Part model, mm, in its own coordinate system. A direction names the side the tool comes from. Give positions to 0.01 mm unless a question says otherwise; leave off trailing zeros. Write each loop counter-clockwise with the first axis right and the second up, starting at its lowest first coordinate (ties: lowest second). Pieces come first, ordered by that corner, then holes. Notation, with made-up numbers: M 20.5,33 L 69.5,33 A20 cw 69.5,61 Z; hole C -29,-19 d1. An arc over 180 degrees is marked long. Use CSV: the item, a comma, the result in double quotes. Start each with the question number.
Item 1: Pin check, flat tips, straight feed: pin 1 (18 mm diameter, centred on x = 20.5, z = -3.5, fed in from +Y); pin 2 (4 mm diameter, centred on x = -7, z = -0.5, fed in from +Y); pin 3 (1.7 mm diameter, centred on x = -14.1, z = -4.95, fed in from +Y); pin 4 (10 mm diameter, centred on y = 17.5, z = -0.5, fed in from -X). Stop position of each tip, or through.
Item 2: Mould opens along Z. For faces 1 (the flat face through (39, 11, 23.5)), 2 (the flat face through (16, 11, -11.25)), 3 (the cylindrical face through (-23.494, 3.36, -0.517)) say: released by +Z, released by -Z, zero draft, split by the parting line, or undercut.
Item 3: Cut at B-B (y = 14.25). List the corners of the cut face in (x, z), then the cut area to 3 significant figures.
Item 4: Which spindle directions (+Z, -Z, +X, -X, +Y, -Y) get a long thin tool onto all of the face, cutting with end or side? Do faces 4 (the flat face through (16, 11, 11.25)), 5 (the cylindrical face through (35.57, 1.48, 3.97)). Say none if no direction does.
Item 5: Cut at C-C (z = -2.5). List the corners of the cut face in (x, y), then the cut area to 3 significant figures.
Item 6: Cut at A-A (x = 34.5). List the corners of the cut face in (y, z), then the cut area to 3 significant figures.
Item 7: Cut at D-D (y = 8.75). List the corners of the cut face in (x, z).
Item 8: Drill centre lines: line 1 (Z direction, x = 34.5, y = 1.25); line 2 (Z direction, x = 30, y = 15.25); line 3 (Y direction, x = 3.5, z = 7). Where is each one in solid material? Low to high. Write a range as [from, to].
from build123d import *

# Parameters (mm, degrees)
SKETCH1_R               = 23.5
SKETCH1_W               = 80
SKETCH1_H               = 47
BOSS_EXTRUDE1_DEPTH     = 23
SKETCH3_W               = 56
SKETCH3_H               = 22.5
CUT_EXTRUDE1_DEPTH      = 20
CUT_EXTRUDE2_DEPTH      = 48
M3_5X0_6_TAPPED_HOLE1_D = 2.9


with BuildPart() as part:
    # Sketch1 → Boss-Extrude1 (new body)
    with BuildSketch(Plane(origin=(0, 0, 0), x_dir=(1, 0, 0), z_dir=(0, 1, 0))):
        Circle(SKETCH1_R)
        with Locations((40, 0)):
            Rectangle(SKETCH1_W, SKETCH1_H)
    extrude(amount=BOSS_EXTRUDE1_DEPTH)

    # Sketch3 → Cut-Extrude1 (cut)
    with BuildSketch(Plane(origin=(0, 23, 0), x_dir=(1, 0, 0), z_dir=(0, 1, 0))):
        with Locations((10.2, 0)):
            Rectangle(SKETCH3_W, SKETCH3_H)
    extrude(amount=-CUT_EXTRUDE1_DEPTH, mode=Mode.SUBTRACT)

    # Sketch4 → Cut-Extrude2 (cut, through all)
    with BuildSketch(Plane.XY.offset(23.5)):
        with BuildLine():
            Line((0, 23), (29.574214856, 23))
            ThreePointArc((29.574214856, 23), (13.980947767, 19.955758133), (0, 12.409203517))
            ThreePointArc((0, 12.409203517), (-11.118700592, 6.831963759), (-23.5, 5.634244617))
            Line((-23.5, 5.634244617), (-23.5, 23))
            Line((-23.5, 23), (0, 23))
        make_face()
    extrude(amount=-CUT_EXTRUDE2_DEPTH, mode=Mode.SUBTRACT)

    # M3.5x0.6 Tapped Hole1 (through all)
    with Locations(Plane(origin=(0, 3, 0), x_dir=(1, 0, 0), z_dir=(0, 1, 0))):
        with Locations((-14.100375238, 4.953237367), (-14.100375238, -4.956255047), (34.5, -4.95), (34.5, 4.953237367)):
            Hole(M3_5X0_6_TAPPED_HOLE1_D / 2)


solid = part.part
Worked answers:
1,pin 1,"stops at y = 22.62"
1,pin 2,"stops at y = 3"
1,pin 3,"passes through"
1,pin 4,"stops at x = 38.2"
2,face 1,"released by +Z"
2,face 2,"undercut"
2,face 3,"split by the parting line"
3,outline,"M 2.6,-23.5 L 80,-23.5 L 80,23.5 L 2.6,23.5 L 2.6,11.25 L 38.2,11.25 L 38.2,-11.25 L 2.6,-11.25 Z"
3,area,"2,840 mm^2"
4,face 4,"+Y"
4,face 5,"+Y, -Y"
5,outline,"M -23.37,0 L 80,0 L 80,23 L 38.2,23 L 38.2,3 L -17.8,3 L -17.8,5.61 A33.95 cw -23.37,5.62 Z"
5,area,"1,160 mm^2"
6,outline,"M 0,-23.5 L 23,-23.5 L 23,-11.25 L 3,-11.25 L 3,-6.4 L 0,-6.4 Z; M 0,-3.5 L 3,-3.5 L 3,3.5 L 0,3.5 Z; M 0,6.4 L 3,6.4 L 3,11.25 L 23,11.25 L 23,23.5 L 0,23.5 Z"
6,area,"614 mm^2"
7,outline,"M -6.04,-22.71 A23.5 ccw 0,-23.5 L 80,-23.5 L 80,23.5 L 0,23.5 A23.5 ccw -6.04,22.71 L -6.04,11.25 L 38.2,11.25 L 38.2,-11.25 L -6.04,-11.25 Z"
8,line 1,"z = [-23.5, -6.4], [-3.5, 3.5], [6.4, 23.5]"
8,line 2,"z = [-23.5, -11.25], [11.25, 23.5]"
8,line 3,"y = [0, 3]"
